Can you work these out from the model? Positions are in its coordinate system, mm. Face numbers are marked on the shaded views. A direction names the side the tool comes from. Round coordinates to 2 decimals unless told otherwise and drop trailing zeros. Write each loop counter-clockwise with the first axis right and the second up, starting at its lowest first coordinate (ties: lowest second). Pieces come first, ordered by that corner, then holes. Notation, with made-up numbers: (-9, 1) - (33, 1) arc R30 cw to (33, 23) - close; hole circle Ø4 at (42.5, -34.5). An arc over 180 degrees is marked (long way). One line per item, written item: value. Start each with the question number.
(1) If I drill on L1, parallel to X at y = 2.65, z = -18.5; L2, parallel to X at y = 4.75, z = 5; L3, parallel to Z at x = 13, y = 3.45, over which ranges is the centre line in solid material (lowest first)? Write a range as from..to.
(2) I want a section at C-C on y = 8.25. Give the number of separate pieces and of enclosed holes in the cut face, plus the area to 3 significant figures.
(3) I'm going to push flat-ended pins straight in: pin 1 Ø4 at (y, z) = (9, -5.5) entering from -X; pin 2 Ø19.5 at (x, z) = (-15.5, -2) entering from +Y; pin 3 Ø3 at (y, z) = (2, 34.5) entering from -X. Where does each tip first touch, or does it pass through?
(4) I want a section at B-B on x = 13. List the corners of the cut face in (y, z) for me.
(5) On a 3-axis mill with a long thin cutter (end or side, diameter ignored), from which of +Z, -Z, +X, -X, +Y, -Y can I reach the whole of each face in a straight line? I mean the marked faces 3 and 4. Say none if no direction works.
(6) Thinking about a two-plate mould opening in Z: for the marked faces 1 and 2, which applies, +Z half, -Z half, draft (parallel to the pull), parting line (faces both ways), or undercut?
(7) I want a section at A-A on x = -60.5. List the corners of the cut face in (y, z) for me, plus the area to 3 significant figures.
from build123d import *

# Parameters (mm, degrees)
SKETCH1_W               = 200
SKETCH1_H               = 150
SKETCH1_R               = 6
SKETCH1_R_2             = 13.5
SKETCH1_R_3             = 2
SKETCH1_R_4             = 2.5
BOSS_EXTRUDE1_DEPTH     = 4
SKETCH3_W               = 200
SKETCH3_H               = 150
BOSS_EXTRUDE2_DEPTH     = 8.25
SKETCH6_R               = 5.4
CUT_EXTRUDE2_DEPTH      = 8.25
FILLET1_R               = 2.5
FILLET2_R               = 5
SKETCH2_R               = 4.4
SKETCH2_R_2             = 5.4
CUT_EXTRUDE1_DEPTH      = 2
CUT_EXTRUDE3_DEPTH      = 126.598815828
CUT_EXTRUDE3_DEPTH_BACK = 126.598815828
SKETCH8_R               = 3
SKETCH9_R               = 5.85
CUT_EXTRUDE4_DEPTH      = 6.5
CUT_EXTRUDE5_DEPTH      = 126.598815818
CUT_EXTRUDE5_DEPTH_BACK = 126.598815818
SKETCH12_OUTSIDE_W      = 252.06
SKETCH12_OUTSIDE_H      = 202.06


with BuildPart() as part:
    # Sketch1 → Boss-Extrude1 (new body)
    with BuildSketch(Plane(origin=(0, 0, 0), x_dir=(1, 0, 0), z_dir=(0, 1, 0))):
        Rectangle(SKETCH1_W, SKETCH1_H)
        with Locations(Location((35.5, 0, 0), (0, 0, 270))):
            Circle(SKETCH1_R, mode=Mode.SUBTRACT)
        with Locations(Location((-35.5, 0, 0), (0, 0, 270))):
            Circle(SKETCH1_R_2, mode=Mode.SUBTRACT)
        with Locations(Location((-60.5, 0, 0), (0, 0, 270))):
            Circle(SKETCH1_R_3, mode=Mode.SUBTRACT)
        with Locations(Location((-35.5, 25, 0), (0, 0, 270))):
            Circle(SKETCH1_R_3, mode=Mode.SUBTRACT)
        with Locations(Location((-10.5, 0, 0), (0, 0, 270))):
            Circle(SKETCH1_R_3, mode=Mode.SUBTRACT)
        with Locations(Location((-35.5, -25, 0), (0, 0, 270))):
            Circle(SKETCH1_R_3, mode=Mode.SUBTRACT)
        with Locations(Location((35.5, 18.5, 0), (0, 0, 270))):
            Circle(SKETCH1_R_4, mode=Mode.SUBTRACT)
        with Locations(Location((35.5, -18.5, 0), (0, 0, 90))):
            Circle(SKETCH1_R_4, mode=Mode.SUBTRACT)
        Polygon((4.517711304, -15.136418767), (0.159242352, 0.258507293), (4.681501882, 1.538807548), (9.039970835, -13.856118512), (9.584779454, -15.78048427), (5.062519924, -17.060784524), align=None, mode=Mode.SUBTRACT)
    extrude(amount=BOSS_EXTRUDE1_DEPTH)

    # Sketch3 → Boss-Extrude2 (add)
    with BuildSketch(Plane(origin=(0, 4, 0), x_dir=(1, 0, 0), z_dir=(0, 1, 0))):
        Rectangle(SKETCH3_W, SKETCH3_H)
        with BuildLine():
            Line((-26.573943662, 31.250208291), (39.070422535, 12.500083317))
            ThreePointArc((39.070422535, 12.500083317), (48.5, 0), (39.070422535, -12.500083317))
            Line((39.070422535, -12.500083317), (-26.573943662, -31.250208291))
            ThreePointArc((-26.573943662, -31.250208291), (-68, 0), (-26.573943662, 31.250208291))
        make_face(mode=Mode.SUBTRACT)
    extrude(amount=BOSS_EXTRUDE2_DEPTH)

    # Sketch6 → Cut-Extrude2 (cut)
    with BuildSketch(Plane(origin=(0, 12.25, 0), x_dir=(1, 0, 0), z_dir=(0, 1, 0))):
        with Locations((35.5, 18.5)):
            Circle(SKETCH6_R)
        with Locations((35.5, -18.5)):
            Circle(SKETCH6_R)
    extrude(amount=-CUT_EXTRUDE2_DEPTH, mode=Mode.SUBTRACT)

    # Fillet1
    # the kernel refuses this fillet: 2.5 mm, written as the material it adds along each edge
    with BuildSketch(Plane(origin=(9.584779454, 0, 15.78048427), x_dir=(-0.9621828787440704, 0, 0.2724043095323078), z_dir=(0, 1, 0)), Plane(origin=(5.062519924, 0, 17.060784524), x_dir=(-0.2724043095323296, 0, -0.9621828787440644), z_dir=(0, 1, 0)), Plane(origin=(4.681501882, 0, -1.538807548), x_dir=(0.2724043095323091, 0, 0.96218287874407), z_dir=(0, 1, 0))) as fillet1_piece_1:
        with BuildLine():
            CenterArc((FILLET1_R, -FILLET1_R), FILLET1_R, 90, 90)
            Line((0, -FILLET1_R), (0, 0))
            Line((0, 0), (FILLET1_R, 0))
        make_face()
    extrude(amount=4)
    with BuildSketch(Plane(origin=(0.159242352, 0, -0.258507293), x_dir=(0.272404309532306, 0, 0.962182878744071), z_dir=(0, 1, 0))) as fillet1_piece_2:
        with BuildLine():
            CenterArc((FILLET1_R, FILLET1_R), FILLET1_R, 180, 90)
            Line((0, FILLET1_R), (0, 0))
            Line((0, 0), (FILLET1_R, 0))
        make_face()
    extrude(amount=4)

    # Fillet2
    fillet2_edges = [part.edges().sort_by_distance(p)[0] for p in [
        (31.784909874, 8.125, 14.581058133),
        (36.584743308, 8.125, 13.210072594),
        (36.584743308, 8.125, -13.210072594),
        (31.784909874, 8.125, -14.581058133),
    ]]
    fillet(fillet2_edges, radius=FILLET2_R)

    # Sketch2 → Cut-Extrude1 (cut)
    with BuildSketch(Plane(origin=(0, 4, 0), x_dir=(1, 0, 0), z_dir=(0, 1, 0))):
        with Locations(Location((-35.5, 25, 0), (0, 0, 270))):
            Circle(SKETCH2_R)
        with Locations(Location((-10.5, 0, 0), (0, 0, 270))):
            Circle(SKETCH2_R)
        with Locations(Location((-35.5, -25, 0), (0, 0, 270))):
            Circle(SKETCH2_R)
        with Locations(Location((-60.5, 0, 0), (0, 0, 270))):
            Circle(SKETCH2_R)
        with Locations(Location((35.5, 18.5, 0), (0, 0, 270))):
            Circle(SKETCH2_R_2)
        with Locations(Location((35.5, -18.5, 0), (0, 0, 197.105868404))):
            Circle(SKETCH2_R_2)
    extrude(amount=-CUT_EXTRUDE1_DEPTH, mode=Mode.SUBTRACT)

    # Sketch8 → Cut-Extrude3 (cut, two sides: drawn at the far end of the back side and taken through both)
    with BuildSketch(Plane.XZ.offset(-CUT_EXTRUDE3_DEPTH_BACK)):
        with Locations(Location((-80.25, 0, 0), (0, 0, 270))):
            Circle(SKETCH8_R)
        with Locations(Location((58, 15, 0), (0, 0, 270))):
            Circle(SKETCH8_R)
        with Locations(Location((58, -15, 0), (0, 0, 270))):
            Circle(SKETCH8_R)
        with Locations(Location((13, 33.75, 0), (0, 0, 270))):
            Circle(SKETCH8_R)
        with Locations(Location((13, -33.75, 0), (0, 0, 270))):
            Circle(SKETCH8_R)
    extrude(amount=CUT_EXTRUDE3_DEPTH + CUT_EXTRUDE3_DEPTH_BACK, mode=Mode.SUBTRACT)

    # Sketch9 → Cut-Extrude4 (cut)
    with BuildSketch(Plane(origin=(0, 12.25, 0), x_dir=(1, 0, 0), z_dir=(0, 1, 0))):
        with Locations(Location((13, 33.75, 0), (0, 0, 270))):
            Circle(SKETCH9_R)
        with Locations(Location((58, 15, 0), (0, 0, 270))):
            Circle(SKETCH9_R)
        with Locations(Location((58, -15, 0), (0, 0, 270))):
            Circle(SKETCH9_R)
        with Locations(Location((13, -33.75, 0), (0, 0, 270))):
            Circle(SKETCH9_R)
        with Locations(Location((-80.25, 0, 0), (0, 0, 270))):
            Circle(SKETCH9_R)
    extrude(amount=-CUT_EXTRUDE4_DEPTH, mode=Mode.SUBTRACT)

    # Sketch12 outside → Cut-Extrude5 (cut, two sides: drawn at the far end of the back side and taken through both)
    with BuildSketch(Plane(origin=(0, 12.25, 0), x_dir=(1, 0, 0), z_dir=(0, 1, 0)).offset(-CUT_EXTRUDE5_DEPTH_BACK)):
        Rectangle(SKETCH12_OUTSIDE_W, SKETCH12_OUTSIDE_H)
        with BuildLine():
            Line((3.977446341, 27.723722089), (-25.200704225, 36.057932644))
            ThreePointArc((-25.200704225, 36.057932644), (-55.024015532, 32.016602217), (-72.271955307, 7.353455166))
            ThreePointArc((-72.271955307, 7.353455166), (-91.1, 0), (-72.271955307, -7.353455166))
            ThreePointArc((-72.271955307, -7.353455166), (-55.024015532, -32.016602217), (-25.200704225, -36.057932644))
            Line((-25.200704225, -36.057932644), (3.977446341, -27.723722089))
            ThreePointArc((3.977446341, -27.723722089), (15.979929577, -44.182761845), (17.478470354, -23.867398961))
            Line((17.478470354, -23.867398961), (25.56006591, -21.559037476))
            ThreePointArc((25.56006591, -21.559037476), (38.738291539, -28.382988815), (45.322811211, -15.083513514))
            ThreePointArc((45.322811211, -15.083513514), (46.302433123, -14.398174837), (47.234399361, -13.649317625))
            ThreePointArc((47.234399361, -13.649317625), (67.027745694, -21.018497129), (52.612600639, -5.582015708))
            ThreePointArc((52.612600639, -5.582015708), (53.5, 0), (52.612600639, 5.582015708))
            ThreePointArc((52.612600639, 5.582015708), (67.027745694, 21.018497129), (47.234399361, 13.649317625))
            ThreePointArc((47.234399361, 13.649317625), (46.302433123, 14.398174837), (45.322811211, 15.083513514))
            ThreePointArc((45.322811211, 15.083513514), (38.738291539, 28.382988815), (25.56006591, 21.559037476))
            Line((25.56006591, 21.559037476), (17.478470354, 23.867398961))
            ThreePointArc((17.478470354, 23.867398961), (15.979929577, 44.182761845), (3.977446341, 27.723722089))
        make_face(mode=Mode.SUBTRACT)
    extrude(amount=CUT_EXTRUDE5_DEPTH + CUT_EXTRUDE5_DEPTH_BACK, mode=Mode.SUBTRACT)


solid = part.part
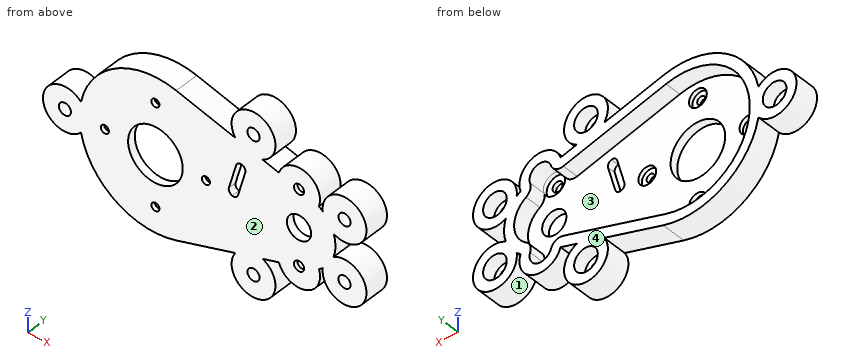
Established:
1. L1: -68.12..30.1, 40.9..45.9, 47.73..68.27
1. L2: -89.88..-67.61, 47.5..52.79, 53.79..62.21
1. L3: -44.6..-36.75, -30.75..30.75, 36.75..44.6
2. separate pieces: 1
2. enclosed holes: 6
2. area: 2,850 mm2
3. pin 1: x = -90.52
3. pin 2: y = 4
3. pin 3: x = -53.31
4. outline: (0, -44.6) - (12.25, -44.6) - (12.25, -39.6) - (5.75, -39.6) - (5.75, -36.75) - (0, -36.75) - close; (0, -30.75) - (5.75, -30.75) - (5.75, -27.9) - (12.25, -27.9) - (12.25, -19.95) - (4, -19.95) - (4, 19.95) - (12.25, 19.95) - (12.25, 27.9) - (5.75, 27.9) - (5.75, 30.75) - (0, 30.75) - close; (0, 36.75) - (5.75, 36.75) - (5.75, 39.6) - (12.25, 39.6) - (12.25, 44.6) - (0, 44.6) - close
5. face 3: +Y
5. face 4: +Z, -Z, +X, -X, +Y
6. face 1: undercut
6. face 2: draft
7. outline: (0, -27.95) - (12.25, -27.95) - (12.25, -20.77) - (4, -20.77) - (4, -4.4) - (2, -4.4) - (2, -2) - (0, -2) - close; (0, 2) - (2, 2) - (2, 4.4) - (4, 4.4) - (4, 20.77) - (12.25, 20.77) - (12.25, 27.95) - (0, 27.95) - close
7. area: 317 mm2
